```python
from build123d import *

# Parameters (mm, degrees)
F0_R     = 75.971248
F0_R_2   = 70.641117
F1_DEPTH = 10.893734
F2_R     = 72.093094
F3_DEPTH = 15.55609
F4_R     = 75.971248
F4_R_2   = 72.087222
F5_DEPTH = 9.329332


with BuildPart() as f1:
    # F0 (on Front) → F1 (new body)
    with BuildSketch(Plane.XZ):
        Circle(F0_R)
        Circle(F0_R_2, mode=Mode.SUBTRACT)
    extrude(amount=F1_DEPTH)

    # F2 (on Front) → F3 (join)
    with BuildSketch(Plane.XZ):
        Circle(F2_R)
    extrude(amount=F3_DEPTH)

    # F4 (on face) → F5 (join)
    with BuildSketch(Plane(origin=(0, 0, 0), x_dir=(-1, 0, 0), z_dir=(0, 1, 0))):
        Circle(F4_R)
        Circle(F4_R_2, mode=Mode.SUBTRACT)
    extrude(amount=F5_DEPTH)


solid = f1.part
```
Could you check a few things on this model? Use its own coordinates, in mm. A direction names the side the tool comes from. Give positions to 0.01 mm unless a question says otherwise; leave off trailing zeros. Loops run counter-clockwise (first coordinate to the right, second up) from the corner with the lowest first, then second, coordinate; pieces in that order, holes last. Notation, with made-up numbers: (83.25, 49) -> (118.25, 49) arc R21 ccw to (118.25, 76) -> close; hole circle Ø11 at (-9, 58). An arc over 180 degrees is marked (long way). Put each result on its own line as item: value.
(1) Imagine slicing it at A-A on x = 0. Write out the boundary of the cut face in (y, z), plus the area to 3 significant figures.
Computed:
outline: (-15.56, -72.09) -> (-10.89, -72.09) -> (-10.89, -75.97) -> (9.33, -75.97) -> (9.33, -72.09) -> (0, -72.09) -> (0, 72.09) -> (9.33, 72.09) -> (9.33, 75.97) -> (-10.89, 75.97) -> (-10.89, 72.09) -> (-15.56, 72.09) -> close
area: 2,400 mm^2
(2) Imagine slicing it at C-C on y = -6.5. Write out the boundary of the cut face in (x, z).
Computed:
outline: circle Ø151.94 at (0, 0)
(3) I'm going to push flat-ended pins straight in: pin 1 Ø6 at (x, y) = (-54.5, 1.5) entering from +Z; pin 2 Ø10 at (y, z) = (-7.5, 38) entering from -X; pin 3 Ø10 at (x, y) = (7, -5) entering from +Z. Where does each tip first touch, or does it pass through?
Computed:
pin 1: z = 55.85
pin 2: x = -68.43
pin 3: z = 75.94
(4) For faces 4 (the face through (-1, -15.556, 1)), 5 (the face through (-68.76, 4.6, 21.65)), which set-ups out of +Z, -Z, +X, -X, +Y, -Y let a thin tool reach every point of the face, with its end or its side?
Computed:
face 4: +Z, -Z, +X, -X, -Y
face 5: +Y
(5) Please list where these lines run through material, in increasing order: probe 1 along Z at (x, y) = (0, 5); probe 2 along Y at (x, z) = (-32, 31); probe 3 along X at (y, z) = (2.5, -11). Write a range as [from, to].
Computed:
probe 1: [-75.97, -72.09], [72.09, 75.97]
probe 2: [-15.56, 0]
probe 3: [-75.17, -71.24], [71.24, 75.17]
(6) Thinking about a two-plate mould opening in Z: for faces 1 (the face through (-57, -10.894, -45)), 2 (the face through (68.764, -13.192, 21.655)), 3 (the face through (-1, 0, 1)), which applies, pulls with the +Z half, pulls with the -Z half, needs draft (parallel to the pull), parting line crosses it, or undercut?
Computed:
face 1: needs draft
face 2: parting line crosses it
face 3: undercut
(7) Imagine slicing it at B-B on z = 0. Write out the boundary of the cut face in (x, y).
Computed:
outline: (-75.97, -10.89) -> (-72.09, -10.89) -> (-72.09, -15.56) -> (72.09, -15.56) -> (72.09, -10.89) -> (75.97, -10.89) -> (75.97, 9.33) -> (72.09, 9.33) -> (72.09, 0) -> (-72.09, 0) -> (-72.09, 9.33) -> (-75.97, 9.33) -> close
